Source: CAD feature listing. Evaluate the final solid. Frame: model axes, mm. Give positions to 0.01 mm unless a question says otherwise; leave off trailing zeros. Order: outer loops, then holes, each group sorted by start corner. A loop starts at its lowest first (then second) coordinate and runs counter-clockwise, first axis right, second up. Notation, with made-up numbers: (80.25, 20) - (115.25, 20) arc R8 cw to (115.25, 25) - close; hole circle Ø6 at (1.25, -25). An arc over 180 degrees is marked (long way). Use CSV: the item, a comma, the result in double quotes.
```python
from build123d import *

# Parameters (mm, degrees)
F0_R     = 2.05
F0_R_2   = 2.5
F0_R_3   = 1.5
F1_DEPTH = 3
F2_R     = 2.05
F3_DEPTH = 25
F5_DEPTH = 25


with BuildPart() as f1:
    # F0 (on Top) → F1 (new body)
    with BuildSketch(Plane.XY):
        Polygon((-64.712085, 0), (0, 0), (-221.649493, 548.601745), (-410, 1160), (-472.782601, 1160), (-278.237843, 528.494797), align=None)
        with Locations((-246.249673, 529.405314)):
            Circle(F0_R, mode=Mode.SUBTRACT)
        with Locations((-253.471547, 550)):
            Circle(F0_R_2, mode=Mode.SUBTRACT)
        with Locations((-261.715064, 576.759006)):
            Circle(F0_R_2, mode=Mode.SUBTRACT)
        with Locations((-125.984579, 178.349417)):
            Circle(F0_R, mode=Mode.SUBTRACT)
        with Locations((-66.047524, 30)):
            Circle(F0_R, mode=Mode.SUBTRACT)
        with Locations((-96.016051, 104.174708)):
            Circle(F0_R, mode=Mode.SUBTRACT)
        with Locations((-62.488111, 74.579486)):
            Circle(F0_R_2, mode=Mode.SUBTRACT)
        with Locations((-28.96017, 44.984264)):
            Circle(F0_R, mode=Mode.SUBTRACT)
        with Locations((-58.928697, 119.158972)):
            Circle(F0_R, mode=Mode.SUBTRACT)
        with Locations((-96.951917, 159.880401)):
            Circle(F0_R_3, mode=Mode.SUBTRACT)
        with Locations((-92.456638, 148.754194)):
            Circle(F0_R_2, mode=Mode.SUBTRACT)
        with Locations((-88.897225, 193.33368)):
            Circle(F0_R, mode=Mode.SUBTRACT)
        with Locations((-192.851205, 397.239467)):
            Circle(F0_R_2, mode=Mode.SUBTRACT)
        with Locations((-197.346484, 408.365674)):
            Circle(F0_R_3, mode=Mode.SUBTRACT)
        with Locations((-214.408113, 450.594686)):
            Circle(F0_R, mode=Mode.SUBTRACT)
        with Locations((-208.584682, 436.181189)):
            Circle(F0_R_2, mode=Mode.SUBTRACT)
        with Locations((-265.248001, 588.227152)):
            Circle(F0_R_3, mode=Mode.SUBTRACT)
        with Locations((-388.900768, 989.612245)):
            Circle(F0_R_2, mode=Mode.SUBTRACT)
        with Locations((-420.402782, 1091.869876)):
            Circle(F0_R, mode=Mode.SUBTRACT)
        with Locations((-412.453676, 1066.066549)):
            Circle(F0_R_2, mode=Mode.SUBTRACT)
    extrude(amount=F1_DEPTH)

    # F2 (on face) → F3 (cut)
    with BuildSketch(Plane.XY.offset(3)):
        with Locations((-252.937843, 490)):
            Circle(F2_R)
        with Locations((-212.937843, 490)):
            Circle(F2_R)
        with Locations((-447.05, 1152)):
            Circle(F2_R)
        with Locations((-417.05, 1152)):
            Circle(F2_R)
        with Locations((-447.05, 1128)):
            Circle(F2_R)
        with Locations((-417.05, 1128)):
            Circle(F2_R)
    extrude(amount=-F3_DEPTH, mode=Mode.SUBTRACT)

    # F4 (on face) → F5 (cut)
    with BuildSketch(Plane.XY.offset(3)):
        Polygon((-460.782601, 1121.047203), (-460.782601, 1160), (-472.782601, 1160), align=None)
    extrude(amount=-F5_DEPTH, mode=Mode.SUBTRACT)


solid = f1.part
```
Item 1: Section B-B on y = 317.5. Return the cut outline in (x, z), then the cut area to 3 significant figures.
Filled in:
outline,"(-192.99, 0) - (-128.28, 0) - (-128.28, 3) - (-192.99, 3) - close"
area,"194 mm2"
Item 2: Section C-C on x = -44. Return the cut outline in (y, z), then the cut area to 3 significant figures.
Filled in:
outline,"(0, 0) - (108.9, 0) - (108.9, 3) - (0, 3) - close"
area,"327 mm2"
Item 3: Material intervals for line 1 (X direction, y = 1128, z = 2.25); line 2 (X direction, y = 393.5, z = 1.7); line 3 (Y direction, x = -88, z = 2.05), sorted ascending. Write a range as from..to.
Filled in:
line 1,"x = -460.78..-449.1, -445..-419.1, -415..-400.14"
line 2,"x = -223.7..-158.98"
line 3,"y = 57.64..191.49, 195.18..217.81"
Item 4: Section A-A on z = 0.9. Count the separate pieces of the cut face and the enclosed holes in it, then the cut area to 3 significant figures.
Filled in:
separate pieces,"1"
enclosed holes,"26"
area,"73,300 mm2"
